from build123d import *

# Parameters (mm, degrees)
BOSS_EXTRUDE1_DEPTH = 49.53
SKETCH2_R           = 1.905
CUT_EXTRUDE1_DEPTH  = 7.239


with BuildPart() as part:
    # Sketch1 → Boss-Extrude1 (new body)
    with BuildSketch(Plane(origin=(0, 0, 0), x_dir=(1, 0, 0), z_dir=(0, 1, 0))):
        with BuildLine():
            Line((0.592937145, 0), (5.122062855, 0))
            ThreePointArc((5.122062855, 0), (5.659328642, 0.119241348), (6.095705772, 0.454574057))
            Line((6.095705772, 0.454574057), (8.222955772, 2.994574057))
            ThreePointArc((8.222955772, 2.994574057), (8.400071506, 4.347265787), (7.249312855, 5.08))
            Line((7.249312855, 5.08), (6.0325, 5.08))
            Line((6.0325, 5.08), (6.0325, 7.239))
            Line((6.0325, 7.239), (-0.3175, 7.239))
            Line((-0.3175, 7.239), (-0.3175, 5.08))
            Line((-0.3175, 5.08), (-1.534312855, 5.08))
            ThreePointArc((-1.534312855, 5.08), (-2.685071506, 4.347265787), (-2.507955772, 2.994574057))
            Line((-2.507955772, 2.994574057), (-0.380705772, 0.454574057))
            ThreePointArc((-0.380705772, 0.454574057), (0.055671358, 0.119241348), (0.592937145, 0))
        make_face()
    extrude(amount=BOSS_EXTRUDE1_DEPTH)

    # Sketch2 → Cut-Extrude1 (cut)
    with BuildSketch(Plane(origin=(0, 0, -7.239), x_dir=(-1, 0, 0), z_dir=(0, 0, -1))):
        with Locations((-2.897477191, 5.715)):
            Circle(SKETCH2_R)
        with Locations((-2.897477191, 26.035)):
            Circle(SKETCH2_R)
    extrude(amount=-CUT_EXTRUDE1_DEPTH, mode=Mode.SUBTRACT)


solid = part.part
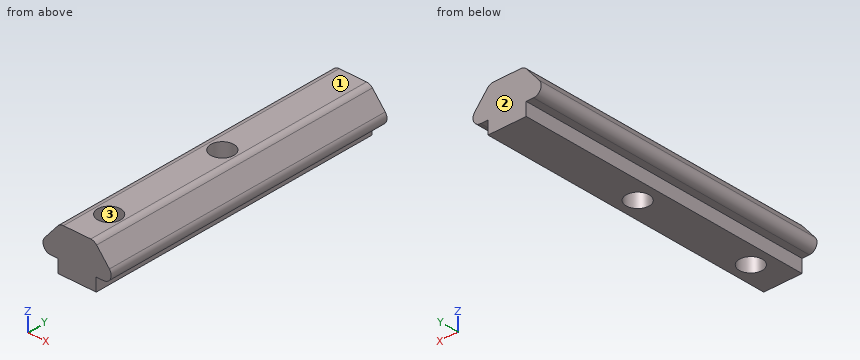
For this review, take the finished solid that the model builds, in its own axes (mm). Face numbers are marked on the shaded views. Round coordinates to 2 decimals unless told otherwise and drop trailing zeros. Loops run counter-clockwise (first coordinate to the right, second up) from the corner with the lowest first, then second, coordinate; pieces in that order, holes last. Notation, with made-up numbers: (53.25, -11.5) - (86.25, -11.5) arc R6 ccw to (86.25, -7.5) - close; hole circle Ø4 at (56.5, 76). An arc over 180 degrees is marked (long way). Answer as CSV lines item,"result".
(1) Consider section D-D on y = 41. Give the boundary of the cut face in (x, z), then the cut area to 3 significant figures.
Checked values:
outline,"(-2.51, -2.99) arc R1.27 ccw to (-1.53, -5.08) - (-0.32, -5.08) - (-0.32, -7.24) - (6.03, -7.24) - (6.03, -5.08) - (7.25, -5.08) arc R1.27 ccw to (8.22, -2.99) - (6.1, -0.45) arc R1.27 ccw to (5.12, 0) - (0.59, 0) arc R1.27 ccw to (-0.38, -0.45) - close"
area,"61.0 mm2"
(2) Insertion check: P1, Ø1, axis at x = 3.5, z = -2.5, coming from the -Y side; P2, Ø2.5, axis at x = 2.9, y = 26.04, coming from the +Z side; P3, Ø0.6, axis at x = 6.5, y = 17.5, coming from the -Z side; P4, Ø1.1, axis at y = 17.5, z = -6.5, coming from the +X side. Each pin has a flat end and moves straight along its axis. Give the tip position at first contact, or say it passes through.
Checked values:
P1,"stops at y = 0"
P2,"passes through"
P3,"stops at z = -5.08"
P4,"stops at x = 6.03"
(3) Consider section B-B on x = 3.75. Give the boundary of the cut face in (y, z), then the cut area to 3 significant figures.
Checked values:
outline,"(0, -7.24) - (4.01, -7.24) - (4.01, 0) - (0, 0) - close; (7.42, -7.24) - (24.33, -7.24) - (24.33, 0) - (7.42, 0) - close; (27.74, -7.24) - (49.53, -7.24) - (49.53, 0) - (27.74, 0) - close"
area,"309 mm2"
(4) Mouldability with a two-part tool opening along Y and no side actions: class the marked faces 1, 2 and 3 as +Y half, -Y half, draft (parallel to the pull), parting line (faces both ways), or undercut.
Checked values:
face 1,"draft"
face 2,"+Y half"
face 3,"undercut"
(5) Consider section A-A on y = 26.5. Give the boundary of the cut face in (x, z).
Checked values:
outline,"(-2.51, -2.99) arc R1.27 ccw to (-1.53, -5.08) - (-0.32, -5.08) - (-0.32, -7.24) - (1.05, -7.24) - (1.05, 0) - (0.59, 0) arc R1.27 ccw to (-0.38, -0.45) - close; (4.74, -7.24) - (6.03, -7.24) - (6.03, -5.08) - (7.25, -5.08) arc R1.27 ccw to (8.22, -2.99) - (6.1, -0.45) arc R1.27 ccw to (5.12, 0) - (4.74, 0) - close"
(6) Wall thickness on line 1 (Y direction, x = 2.75, z = -2); line 2 (Y direction, x = 2.5, z = -2.25); line 3 (X direction, y = 21, z = -6.5): over which ranges is each line inside the solid? List them lowest first.
Checked values:
line 1,"y = 0 to 3.82, 7.61 to 24.14, 27.93 to 49.53"
line 2,"y = 0 to 3.85, 7.58 to 24.17, 27.9 to 49.53"
line 3,"x = -0.32 to 6.03"
(7) Consider section C-C on z = -4.5. Give the boundary of the cut face in (x, y) (3 decimals).
Checked values:
outline,"(-2.601, 0) - (8.316, 0) - (8.316, 49.53) - (-2.601, 49.53) - close; hole circle Ø3.81 at (2.897, 5.715); hole circle Ø3.81 at (2.897, 26.035)"
